```python
from build123d import *

# Parameters (mm, degrees)
SKETCH1_R         = 3.175
SCREWLENGTH_DEPTH = 101.6
SKETCH2_R         = 5.55625
HEAD_DEPTH        = 4
FILLET4_R         = 2


with BuildPart() as part:
    # Sketch1 → Screwlength (new body)
    with BuildSketch(Plane.XY):
        Circle(SKETCH1_R)
    extrude(amount=-SCREWLENGTH_DEPTH)

    # Sketch2 → Head (add)
    with BuildSketch(Plane.XY):
        Circle(SKETCH2_R)
    extrude(amount=HEAD_DEPTH)

    # Fillet4
    fillet4_edges = [part.edges().sort_by_distance(p)[0] for p in [
        (-5.55625, 0, 4),
    ]]
    fillet(fillet4_edges, radius=FILLET4_R)


solid = part.part
```
The listing builds one solid part. Answer for the finished solid, in the listing's coordinates (mm). A direction names the side the tool comes from. Give positions to 0.01 mm unless a question says otherwise; leave off trailing zeros. Order: outer loops, then holes, each group sorted by start corner. A loop starts at its lowest first (then second) coordinate and runs counter-clockwise, first axis right, second up. Notation, with made-up numbers: (-19.5, 62) -> (36.5, 62) arc R24 ccw to (36.5, 91) -> close; hole circle Ø1 at (10.25, -33). An arc over 180 degrees is marked (long way). Answer as CSV lines item,"result". Start each with the question number.
Q1. A cutting plane is placed at C-C (z = -15). Determine the outline of the cut face in (x, y) (3 decimals), then the cut area to 3 significant figures.
Q2. Which of the six approach directions +Z, -Z, +X, -X, +Y, -Y give full straight-line access (tool end or side, diameter ignored) to faces 1 (the flat face through (0, 0, 4)), 2 (the flat face through (2.4, -2.4, 0))?
Q3. Given pin 1 (4 mm diameter, centred on x = 4, y = 1, fed in from -Z); pin 2 (3 mm diameter, centred on x = -0.5, z = -52, fed in from -Y) (3 decimals); pin 3 (1 mm diameter, centred on x = -2, z = -38.5, fed in from -Y); pin 4 (2 mm diameter, centred on x = 3.5, z = -9.5, fed in from -Y), each flat-ended and moving along its own axis, determine where each tip first touches the part or whether it passes through.
Q4. Find the intervals of material crossed by L1, parallel to Z at x = 1.5, y = -3.5; L2, parallel to Y at x = -0.25, z = -75; L3, parallel to Z at x = 2.5, y = 4.5, in increasing order.
Q5. A cutting plane is placed at A-A (x = 0). Determine the outline of the cut face in (y, z) (3 decimals), then the cut area to 3 significant figures.
Results found:
1,outline,"circle Ø6.35 at (0, 0)"
1,area,"31.7 mm2"
2,face 1,"+Z, +X, -X, +Y, -Y"
2,face 2,"-Z"
3,pin 1,"z = -101.6"
3,pin 2,"y = -3.175"
3,pin 3,"y = -2.8"
3,pin 4,"y = -1.96"
4,L1,"0 to 3.98"
4,L2,"-3.17 to 3.17"
4,L3,"0 to 3.21"
5,outline,"(-5.556, 0) -> (-3.175, 0) -> (-3.175, -101.6) -> (3.175, -101.6) -> (3.175, 0) -> (5.556, 0) -> (5.556, 2) arc R2 ccw to (3.556, 4) -> (-3.556, 4) arc R2 ccw to (-5.556, 2) -> close"
5,area,"688 mm2"
